Design review of the part built by this model. Coordinates are the model's own, in mm. A direction names the side the tool comes from. Coordinates: 2 decimals unless noted, no trailing zeros. Loops run counter-clockwise (first coordinate to the right, second up) from the corner with the lowest first, then second, coordinate; pieces in that order, holes last.
Q1. Wall thickness on probe 1 along Y at (x, z) = (63.5, 0.75); probe 2 along Y at (x, z) = (50, 1.75); probe 3 along X at (y, z) = (48, 0.5): over which ranges is each line inside the solid? List them lowest first.
Q2. Add section A-A on y = 36. Give the boundary of the cut face in (x, z) (3 decimals).
Q3. Add section D-D on z = 5.5. Give the boundary of the cut face in (x, y).
Q4. For P1, Ø2.5, axis at x = 75.18, y = 5.51, coming from the +Z side; P2, Ø0.5, axis at x = 47.5, z = 3.5, coming from the -Y side; P3, Ø12, axis at x = 71.5, y = 41.5, coming from the -Z side; P4, Ø2, axis at x = 58, z = 4, coming from the -Y side, all flat-tipped, find the tip position at first contact; note any pin that passes through.
Q5. Machinability: for faces 1 (the face through (46.64, 5.04, 5.59)), 2 (the face through (78.754, 47.131, 4.74)), 3 (the face through (47.82, 28.98, 5.44)), which of the approach directions +Z, -Z, +X, -X, +Y, -Y give a long, thin tool a straight path to every point of the face, cutting with its end or side? Answer none if there is none.
Q6. Add section B-B on x = 56. Give the boundary of the cut face in (y, z) (3 decimals).
Q7. Add section C-C on z = 1.75. Give the boundary of the cut face in (x, y).
Q8. Draft analysis for pull direction Y (two halves, no side actions). For faces 4 (the face through (47, 29, 6.35)), 5 (the face through (62.71, 5.04, 5.59)), 6 (the face through (43.72, 52.315, 3.488)), 7 (the face through (78.52, 28.99, 3.59)), state which applies: released by +Y, released by -Y, zero draft, split by the parting line, or undercut.
```python
from build123d import *
from OCP.BRepFilletAPI import BRepFilletAPI_MakeChamfer

# Parameters (mm, degrees)
MODEL_W             = 40.64000000000001
MODEL_H             = 50.291999999999994
MODEL_R             = 1.3499999999999979
MODEL_R_2           = 1.3499999999999985
MODEL_R_3           = 1.3500000000000056
MODEL_R_4           = 1.3500000000000065
MODEL_W_2           = 32.69080000000003
MODEL_H_2           = 42.690799999999996
BOSS_EXTRUDE1_DEPTH = 3.175
SKETCH1_W           = 32.69080000000003
SKETCH1_H           = 42.690799999999996
SKETCH1_W_2         = 27.828239916797088
SKETCH1_H_2         = 36.340799999999994
BOSS_EXTRUDE2_DEPTH = 3.175
SKETCH2_W           = 39.116000000000014
SKETCH2_H           = 48.768
SKETCH2_W_2         = 32.69080000000003
SKETCH2_H_2         = 42.690799999999996
BOSS_EXTRUDE4_DEPTH = 3.175
FILLET1_R           = 2.54
FILLET2_R           = 2.54
CHAMFER9_SIZE       = 3.175
CHAMFER9_SIZE_2     = 2.858782841
CHAMFER10_SIZE      = 3.175
SKETCH4_R           = 1.3500000000000065
SKETCH4_R_2         = 1.3499999999999979
SKETCH4_R_3         = 1.3499999999999985
SKETCH4_R_4         = 1.3500000000000056
CUT_EXTRUDE1_DEPTH  = 100.03179502787644
CHAMFER11_SIZE      = 0.889
CHAMFER11_SIZE2     = 0.6602398251627483
CHAMFER12_SIZE      = 1.143
CHAMFER12_SIZE2     = 0.9523797142277386
CUT_EXTRUDE2_START  = -3.175
SKETCH5_R           = 2.0955000000000017
SKETCH5_R_2         = 2.095500000000001
CUT_EXTRUDE2_DEPTH  = 3.175


with BuildPart() as part:
    # Model → Boss-Extrude1 (new body)
    with BuildSketch(Plane.XY):
        with Locations((62.55399712221356, 28.695197306808385)):
            Rectangle(MODEL_W, MODEL_H)
        with Locations((44.272200000000005, 47.066199999999995)):
            Circle(MODEL_R, mode=Mode.SUBTRACT)
        with Locations((49.9364, 5.5118)):
            Circle(MODEL_R_2, mode=Mode.SUBTRACT)
        with Locations((75.184, 5.5118)):
            Circle(MODEL_R_3, mode=Mode.SUBTRACT)
        with Locations((80.84819999999999, 47.066199999999995)):
            Circle(MODEL_R_4, mode=Mode.SUBTRACT)
        with Locations((62.55399712221356, 28.69519730680839)):
            Rectangle(MODEL_W_2, MODEL_H_2, mode=Mode.SUBTRACT)
    extrude(amount=BOSS_EXTRUDE1_DEPTH)



with BuildPart() as body_2:
    # Sketch1 → Boss-Extrude2 (new body)
    with BuildSketch(Plane.XY.offset(3.175)):
        with Locations((62.55399712221356, 28.69519730680839)):
            Rectangle(SKETCH1_W, SKETCH1_H)
        with Locations((62.55399712221356, 28.695197306808385)):
            Rectangle(SKETCH1_W_2, SKETCH1_H_2, mode=Mode.SUBTRACT)
    extrude(amount=BOSS_EXTRUDE2_DEPTH)


with BuildPart() as part_1:
    add(part.part)

    add(body_2.part)  # Boss-Extrude4 merges body 2
    # Sketch2 → Boss-Extrude4 (add)
    with BuildSketch(Plane.XY.offset(3.175)):
        with Locations((62.55399712221356, 28.69519730680838)):
            Rectangle(SKETCH2_W, SKETCH2_H)
        with Locations((62.55399712221356, 28.69519730680839)):
            Rectangle(SKETCH2_W_2, SKETCH2_H_2, mode=Mode.SUBTRACT)
    extrude(amount=BOSS_EXTRUDE4_DEPTH)

    # Fillet1
    fillet1_edges = [part_1.edges().sort_by_distance(p)[0] for p in [
        (62.55399712221356, 4.311197306808385, 6.35),
        (62.55399712221356, 53.07919730680838, 6.35),
    ]]
    fillet(fillet1_edges, radius=FILLET1_R)

    # Fillet2
    fillet2_edges = [part_1.edges().sort_by_distance(p)[0] for p in [
        (82.11199712221357, 52.335248531022216, 5.6060512242138305),
        (82.11199712221357, 5.055146082594554, 5.606051224213831),
        (42.99599712221355, 4.311197306808385, 3.4924999999999997),
        (42.99599712221355, 53.07919730680838, 3.4924999999999997),
        (42.99599712221355, 52.33524853102221, 5.606051224213832),
        (42.99599712221355, 5.055146082594553, 5.6060512242138305),
        (42.99599712221355, 28.69519730680838, 6.35),
        (82.11199712221357, 28.695197306808385, 6.35),
        (82.11199712221357, 53.07919730680838, 3.4924999999999997),
        (82.11199712221357, 4.311197306808385, 3.4924999999999997),
    ]]
    fillet(fillet2_edges, radius=FILLET2_R)

    # Chamfer9
    # the kernel refuses this chamfer: 3.175, 2.858782841 mm, written as the material it takes off along each edge
    with BuildSketch(Plane(origin=(48.639877163815015, 46.86559730680839, 3.175), x_dir=(0, 0, 1), z_dir=(0, -1, 0))) as chamfer9_piece_1_section:
        Polygon((CHAMFER9_SIZE, 0), (0, CHAMFER9_SIZE_2), (0, 0), align=None)
    chamfer9_piece_1 = extrude(amount=36.3408, mode=Mode.PRIVATE)
    chamfer9_piece_1 = split(chamfer9_piece_1, bisect_by=Plane(origin=(46.20859712221354, 46.86559730680839, 3.175), z_dir=(1, 0, 0)), keep=Keep.TOP, mode=Mode.PRIVATE)
    add(chamfer9_piece_1, mode=Mode.SUBTRACT)
    with BuildSketch(Plane(origin=(76.4681170806121, 10.524797306808388, 3.175), x_dir=(0, 0, 1), z_dir=(0, 1, 0))) as chamfer9_piece_2_section:
        Polygon((CHAMFER9_SIZE, 0), (0, CHAMFER9_SIZE_2), (0, 0), align=None)
    chamfer9_piece_2 = extrude(amount=36.3408, mode=Mode.PRIVATE)
    chamfer9_piece_2 = split(chamfer9_piece_2, bisect_by=Plane(origin=(78.89939712221357, 10.524797306808388, 3.175), z_dir=(-1, 0, 0)), keep=Keep.TOP, mode=Mode.PRIVATE)
    add(chamfer9_piece_2, mode=Mode.SUBTRACT)

    # Chamfer10
    # the kernel refuses this chamfer: 3.175 mm, written as the material it takes off along each edge
    with BuildSketch(Plane(origin=(46.208597122214, 46.865597306808, 3.175), x_dir=(0, 1.2309e-13, 1), z_dir=(1, 0, 0))) as chamfer10_piece_1_section:
        Polygon((CHAMFER10_SIZE, 0), (3.908e-13, -CHAMFER10_SIZE), (0, 0), align=None)
    chamfer10_piece_1 = extrude(amount=32.690799999999996, mode=Mode.PRIVATE)
    chamfer10_piece_1 = split(chamfer10_piece_1, bisect_by=Plane(origin=(64.4986511687098, 46.865597306808, 19.643438635932224), z_dir=(-0.7431448254361507, 0, -0.6691306064046639)), keep=Keep.TOP, mode=Mode.PRIVATE)
    chamfer10_piece_1 = split(chamfer10_piece_1, bisect_by=Plane(origin=(45.97250261720881, 46.865597306808, 3.387580447169522), z_dir=(0.7431448254361507, 0, -0.6691306064046639)), keep=Keep.TOP, mode=Mode.PRIVATE)
    add(chamfer10_piece_1, mode=Mode.SUBTRACT)
    with BuildSketch(Plane(origin=(78.899397122214, 10.524797306808, 3.175), x_dir=(1.1e-16, -1, 0), z_dir=(-1, -1.1e-16, 0))) as chamfer10_piece_2_section:
        Polygon((CHAMFER10_SIZE, 0), (-3.908e-13, CHAMFER10_SIZE), (0, 0), align=None)
    chamfer10_piece_2 = extrude(amount=32.690799999999996, mode=Mode.PRIVATE)
    chamfer10_piece_2 = split(chamfer10_piece_2, bisect_by=Plane(origin=(79.13549162721864, 10.524797306808, 3.38758044716903), z_dir=(-0.7431448254361507, 0, -0.6691306064046639)), keep=Keep.TOP, mode=Mode.PRIVATE)
    chamfer10_piece_2 = split(chamfer10_piece_2, bisect_by=Plane(origin=(60.609343075717646, 10.524797306808, 19.64343863593272), z_dir=(0.7431448254361507, 0, -0.6691306064046639)), keep=Keep.TOP, mode=Mode.PRIVATE)
    add(chamfer10_piece_2, mode=Mode.SUBTRACT)

    # Sketch4 → Cut-Extrude1 (cut, through all)
    with BuildSketch(Plane(origin=(0, 0, 0), x_dir=(-1, 0, 0), z_dir=(0, 0, -1))):
        with Locations(Location((-80.84819999999999, 47.066199999999995, 0), (0, 0, 19.032198816))):
            Circle(SKETCH4_R)
        with Locations(Location((-44.272200000000005, 47.066199999999995, 0), (0, 0, 19.032198816))):
            Circle(SKETCH4_R_2)
        with Locations(Location((-49.9364, 5.5118, 0), (0, 0, 297.210156983))):
            Circle(SKETCH4_R_3)
        with Locations(Location((-75.184, 5.5118, 0), (0, 0, 297.210156983))):
            Circle(SKETCH4_R_4)
    extrude(amount=-CUT_EXTRUDE1_DEPTH, mode=Mode.SUBTRACT)

    # Chamfer11: one chamfer whose edges measure the first distance from different faces: ONE call of the kernel's chamfer builder (chamfer() names one face for all edges)
    chamfer11_edges_1 = [part_1.edges().sort_by_distance(p)[0] for p in [
        (62.55399712221356, 50.04059730680839, 3.175),
    ]]
    chamfer11_side_1 = [part_1.faces().sort_by_distance(p)[0] for p in [
        (62.55399712221734, 48.49951336002211, 4.716083946785889),
    ]]
    chamfer11_edges_2 = [part_1.edges().sort_by_distance(p)[0] for p in [
        (62.55399712221356, 7.349797306808389, 3.175),
    ]]
    chamfer11_side_2 = [part_1.faces().sort_by_distance(p)[0] for p in [
        (62.553997122213964, 8.890881253594266, 4.716083946786265),
    ]]
    chamfer11 = BRepFilletAPI_MakeChamfer(part_1.part.solid().wrapped)
    for e in chamfer11_edges_1:
        chamfer11.Add(CHAMFER11_SIZE, CHAMFER11_SIZE2, e.wrapped, chamfer11_side_1[0].wrapped)  # the first distance lies on this face
    for e in chamfer11_edges_2:
        chamfer11.Add(CHAMFER11_SIZE, CHAMFER11_SIZE2, e.wrapped, chamfer11_side_2[0].wrapped)  # the first distance lies on this face
    add(Compound.cast(chamfer11.Shape()), mode=Mode.REPLACE)

    # Chamfer12: one chamfer whose edges measure the first distance from different faces: ONE call of the kernel's chamfer builder (chamfer() names one face for all edges)
    chamfer12_edges_1 = [part_1.edges().sort_by_distance(p)[0] for p in [
        (46.208597122213995, 28.695197306810893, 3.6497899590838045),
    ]]
    chamfer12_side_1 = [part_1.faces().sort_by_distance(p)[0] for p in [
        (47.396342466238764, 28.695197306818734, 4.9689148024186895),
    ]]
    chamfer12_edges_2 = [part_1.edges().sort_by_distance(p)[0] for p in [
        (78.899397122214, 28.695197306805508, 3.6497899590828133),
    ]]
    chamfer12_side_2 = [part_1.faces().sort_by_distance(p)[0] for p in [
        (77.71165177818875, 28.695197306797276, 4.96891480241812),
    ]]
    chamfer12 = BRepFilletAPI_MakeChamfer(part_1.part.solid().wrapped)
    for e in chamfer12_edges_1:
        chamfer12.Add(CHAMFER12_SIZE, CHAMFER12_SIZE2, e.wrapped, chamfer12_side_1[0].wrapped)  # the first distance lies on this face
    for e in chamfer12_edges_2:
        chamfer12.Add(CHAMFER12_SIZE, CHAMFER12_SIZE2, e.wrapped, chamfer12_side_2[0].wrapped)  # the first distance lies on this face
    add(Compound.cast(chamfer12.Shape()), mode=Mode.REPLACE)

    # Sketch5 → Cut-Extrude2 (cut)
    with BuildSketch(Plane.XY.offset(6.35).offset(CUT_EXTRUDE2_START)):
        with Locations((44.272200000000005, 47.066199999999995)):
            Circle(SKETCH5_R)
        with Locations((80.84819999999999, 47.066199999999995)):
            Circle(SKETCH5_R)
        with Locations((75.184, 5.5118)):
            Circle(SKETCH5_R_2)
        with Locations((49.9364, 5.5118)):
            Circle(SKETCH5_R_2)
    extrude(amount=CUT_EXTRUDE2_DEPTH, mode=Mode.SUBTRACT)


solid = part_1.part
```
Entries:
1. probe 1: y = 3.55 to 7.35, 50.04 to 53.84
1. probe 2: y = 3.55 to 4.16, 6.86 to 7.35, 50.04 to 53.84
1. probe 3: x = 42.23 to 43.3, 45.25 to 46.21, 78.9 to 79.87, 81.82 to 82.87
2. outline: (42.234, 0) - (46.209, 0) - (46.209, 2.697) - (46.973, 4.499) - (48.64, 6.35) - (45.536, 6.35) arc R2.54 ccw to (42.996, 3.81) - (42.996, 3.175) - (42.234, 3.175) - close; (76.468, 6.35) - (78.135, 4.499) - (78.899, 2.697) - (78.899, 0) - (82.874, 0) - (82.874, 3.175) - (82.112, 3.175) - (82.112, 3.81) arc R2.54 ccw to (79.572, 6.35) - close
3. outline: (43.64, 6.85) arc R1.9 ccw to (45.54, 4.96) - (47.92, 4.96) arc R2.1 cw (long way) to (51.96, 4.96) - (73.16, 4.96) arc R2.1 cw (long way) to (77.2, 4.96) - (79.57, 4.96) arc R1.9 ccw to (81.47, 6.85) - (81.47, 45.06) arc R2.1 cw (long way) to (81.47, 49.07) - (81.47, 50.54) arc R1.9 ccw to (79.57, 52.44) - (45.54, 52.44) arc R1.9 ccw to (43.64, 50.54) - (43.64, 49.06) arc R2.1 cw (long way) to (43.64, 45.07) - close; hole (47.87, 9.67) - (77.23, 9.67) - (77.23, 47.72) - (47.87, 47.72) - close
4. P1: passes through
4. P2: stops at y = 4.31
4. P3: stops at z = 5.2
4. P4: stops at y = 3.55
5. face 1: +Z, +X, -X, -Y
5. face 2: +Z
5. face 3: -Z
6. outline: (3.549, 0) - (7.35, 0) - (7.35, 2.515) - (7.978, 3.804) - (10.525, 6.35) - (6.851, 6.35) arc R2.54 ccw to (4.311, 3.81) - (4.311, 3.175) - (3.549, 3.175) - close; (46.866, 6.35) - (49.412, 3.804) - (50.041, 2.515) - (50.041, 0) - (53.841, 0) - (53.841, 3.175) - (53.079, 3.175) - (53.079, 3.81) arc R2.54 ccw to (50.539, 6.35) - close
7. outline: (42.23, 3.55) - (82.87, 3.55) - (82.87, 53.84) - (42.23, 53.84) - close; hole circle Ø2.7 at (44.27, 47.07); hole (46.21, 7.35) - (78.9, 7.35) - (78.9, 50.04) - (46.21, 50.04) - close; hole circle Ø2.7 at (49.94, 5.51); hole circle Ø2.7 at (75.18, 5.51); hole circle Ø2.7 at (80.85, 47.07)
8. face 4: zero draft
8. face 5: released by -Y
8. face 6: released by +Y
8. face 7: undercut
